Verification items for the finished model (mm, model axes). A direction names the side the tool comes from. Coordinates: 2 decimals unless noted, no trailing zeros. Order: outer loops, then holes, each group sorted by start corner. A loop starts at its lowest first (then second) coordinate and runs counter-clockwise, first axis right, second up. Notation, with made-up numbers: (14, 85.25) -> (56, 85.25) arc R15 cw to (56, 98.25) -> close; hole circle Ø6 at (-2.5, -18.5). An arc over 180 degrees is marked (long way). Answer as CSV lines item,"result".
```python
from build123d import *

# Parameters (mm, degrees)
F0_W     = 600
F0_H     = 400
F1_DEPTH = 25
F2_SIZE  = 5
F3_W     = 36.971099
F3_H     = 7
F4_DEPTH = 1000


with BuildPart() as f1:
    # F0 (on Front) → F1 (new body)
    with BuildSketch(Plane.XZ):
        with Locations((-14921.775502, 182.368167)):
            Rectangle(F0_W, F0_H)
    extrude(amount=F1_DEPTH)

    # F2
    f2_edges = [f1.edges().sort_by_distance(p)[0] for p in [
        (-14921.775502, -25, -17.631833),
    ]]
    chamfer(f2_edges, length=F2_SIZE)

    # F3 (on face) → F4 (cut)
    with BuildSketch(Plane(origin=(-15221.775502, 0, 0), x_dir=(0, -1, 0), z_dir=(-1, 0, 0))):
        with Locations((26.485549, 363.868167)):
            Rectangle(F3_W, F3_H)
    extrude(amount=-F4_DEPTH, mode=Mode.SUBTRACT)


solid = f1.part
```
Item 1: Section check A-A, the plane y = -16. Record the boundary of the cut face in (x, z), plus the area to 3 significant figures.
Answer list:
outline,"(-15221.78, -17.63) -> (-14621.78, -17.63) -> (-14621.78, 360.37) -> (-15221.78, 360.37) -> close; (-15221.78, 367.37) -> (-14621.78, 367.37) -> (-14621.78, 382.37) -> (-15221.78, 382.37) -> close"
area,"236,000 mm2"
Item 2: Depth check by flat-ended pin: pin 1 Ø3.5 at (x, z) = (-14918, 363.5) entering from -Y. Enter the tip coordinate at first touch or a pass-through.
Answer list:
pin 1,"y = -8"
Item 3: Thickness scan on line 1 (Z direction, x = -14729, y = -9). Record the ranges inside material, lowest first.
Answer list:
line 1,"-17.63 to 360.37, 367.37 to 382.37"
Item 4: Release check for a two-part mould opening along Z. For faces 1 (the flat face through (-14926, -16, 367.368)), 2 (the flat face through (-14926, -12, 382.368)), 3 (the flat face through (-14621.776, -12, 180)) record: +Z half, -Z half, draft (parallel to the pull), parting line (faces both ways), or undercut.
Answer list:
face 1,"undercut"
face 2,"+Z half"
face 3,"draft"
Item 5: Tool access check on faces 4 (the flat face through (-14926, -16, 360.368)), 5 (the flat face through (-14926, -25, 176)). Record the directions out of +Z, -Z, +X, -X, +Y, -Y that give a thin tool (end or side, any length) a straight path to the whole face; none if there is none.
Answer list:
face 4,"+X, -X, -Y"
face 5,"+Z, -Z, +X, -X, -Y"
